Geometry check sheet. Reference: the model listing, model coordinates, mm. A direction names the side the tool comes from. Round coordinates to 2 decimals unless told otherwise and drop trailing zeros. Write each loop counter-clockwise with the first axis right and the second up, starting at its lowest first coordinate (ties: lowest second). Pieces come first, ordered by that corner, then holes. Notation, with made-up numbers: M 58,-15.5 L 67,-15.5 A21 cw 67,22.5 Z; hole C -32.5,53.25 d10. An arc over 180 degrees is marked long. Use a Markdown table: item, result.
```python
from build123d import *

# Parameters (mm, degrees)
ESQUISSE1_W             = 230
ESQUISSE1_H             = 270
BOSS_EXTRU_2_DEPTH      = 2.5
ENL_V_MAT_EXTRU_1_REACH = 405.102
ESQUISSE4_W             = 210
ESQUISSE4_H             = 23
ESQUISSE5_R             = 2
ENL_V_MAT_EXTRU_2_DEPTH = 2.5
ESQUISSE6_W             = 35
ESQUISSE6_H             = 8
ESQUISSE6_W_2           = 115
ESQUISSE6_H_2           = 25
ENL_V_MAT_EXTRU_3_DEPTH = 2.5
ESQUISSE7_W             = 29
ESQUISSE7_H             = 13
ENL_V_MAT_EXTRU_4_DEPTH = 2.5
ESQUISSE8_W             = 160
ESQUISSE8_H             = 2.5
BOSS_EXTRU_3_DEPTH      = 8
ESQUISSE9_R             = 2
ENL_V_MAT_EXTRU_5_DEPTH = 404.231037827
ESQUISSE11_R            = 2
ENL_V_MAT_EXTRU_6_DEPTH = 404.231037827


with BuildPart() as part:
    # Esquisse1 → Boss.-Extru.2 (new body)
    with BuildSketch(Plane.XY.offset(25)):
        with Locations((-102.459507472, 204.405925813)):
            Rectangle(ESQUISSE1_W, ESQUISSE1_H)
    extrude(amount=BOSS_EXTRU_2_DEPTH)

    # Esquisse4 → Enlèv. mat.-Extru.1 (cut, up to next)
    with BuildSketch(Plane.XY.offset(27.5), mode=Mode.PRIVATE) as enl_v_mat_extru_1_sk1:
        with Locations((-102.459507472, 87.905925813)):
            Rectangle(ESQUISSE4_W, ESQUISSE4_H)
    enl_v_mat_extru_1_tool1 = extrude(enl_v_mat_extru_1_sk1.sketch, amount=-ENL_V_MAT_EXTRU_1_REACH, mode=Mode.PRIVATE) & part.part
    add(enl_v_mat_extru_1_tool1.solids().sort_by_distance((-102.459507, 87.905926, 27.5))[0], mode=Mode.SUBTRACT)

    # Esquisse5 → Enlèv. mat.-Extru.2 (cut)
    with BuildSketch(Plane.XY.offset(27.5)):
        with Locations((-213.459507472, 73.405925813)):
            Circle(ESQUISSE5_R)
        with Locations((8.540492528, 73.405925813)):
            Circle(ESQUISSE5_R)
    extrude(amount=-ENL_V_MAT_EXTRU_2_DEPTH, mode=Mode.SUBTRACT)

    # Esquisse6 → Enlèv. mat.-Extru.3 (cut)
    with BuildSketch(Plane.XY.offset(27.5)):
        with Locations((-168.959507472, 249.405925813)):
            Rectangle(ESQUISSE6_W, ESQUISSE6_H)
        with Locations((-68.959507472, 240.905925813)):
            Rectangle(ESQUISSE6_W_2, ESQUISSE6_H_2)
    extrude(amount=-ENL_V_MAT_EXTRU_3_DEPTH, mode=Mode.SUBTRACT)

    # Esquisse7 → Enlèv. mat.-Extru.4 (cut)
    with BuildSketch(Plane.XY.offset(27.5)):
        with Locations((-131.959507472, 218.905925813)):
            Rectangle(ESQUISSE7_W, ESQUISSE7_H)
        with Locations((-183.959507472, 218.905925813)):
            Rectangle(ESQUISSE7_W, ESQUISSE7_H)
        with Locations((-79.959507472, 218.905925813)):
            Rectangle(ESQUISSE7_W, ESQUISSE7_H)
        with Locations((-27.959507472, 218.905925813)):
            Rectangle(ESQUISSE7_W, ESQUISSE7_H)
        with Locations((-131.959507472, 188.905925813)):
            Rectangle(ESQUISSE7_W, ESQUISSE7_H)
        with Locations((-79.959507472, 188.905925813)):
            Rectangle(ESQUISSE7_W, ESQUISSE7_H)
        with Locations((-27.959507472, 188.905925813)):
            Rectangle(ESQUISSE7_W, ESQUISSE7_H)
        with Locations((-131.959507472, 158.905925813)):
            Rectangle(ESQUISSE7_W, ESQUISSE7_H)
        with Locations((-79.959507472, 158.905925813)):
            Rectangle(ESQUISSE7_W, ESQUISSE7_H)
        with Locations((-27.959507472, 158.905925813)):
            Rectangle(ESQUISSE7_W, ESQUISSE7_H)
        with Locations((-131.959507472, 128.905925813)):
            Rectangle(ESQUISSE7_W, ESQUISSE7_H)
        with Locations((-79.959507472, 128.905925813)):
            Rectangle(ESQUISSE7_W, ESQUISSE7_H)
        with Locations((-27.959507472, 128.905925813)):
            Rectangle(ESQUISSE7_W, ESQUISSE7_H)
        with Locations((-183.959507472, 188.905925813)):
            Rectangle(ESQUISSE7_W, ESQUISSE7_H)
        with Locations((-183.959507472, 158.905925813)):
            Rectangle(ESQUISSE7_W, ESQUISSE7_H)
        with Locations((-183.959507472, 128.905925813)):
            Rectangle(ESQUISSE7_W, ESQUISSE7_H)
    extrude(amount=-ENL_V_MAT_EXTRU_4_DEPTH, mode=Mode.SUBTRACT)

    # Esquisse8 → Boss.-Extru.3 (add)
    with BuildSketch(Plane(origin=(0, 0, 25), x_dir=(-1, 0, 0), z_dir=(0, 0, -1))):
        with Locations((114.330010258, 199.655925813)):
            Rectangle(ESQUISSE8_W, ESQUISSE8_H)
    extrude(amount=BOSS_EXTRU_3_DEPTH)

    # Esquisse9 → Enlèv. mat.-Extru.5 (cut, through all)
    with BuildSketch(Plane.XY.offset(27.5)):
        with Locations((-209.959507472, 265.405925813)):
            Circle(ESQUISSE9_R)
    extrude(amount=-ENL_V_MAT_EXTRU_5_DEPTH, mode=Mode.SUBTRACT)

    # Esquisse11 → Enlèv. mat.-Extru.6 (cut, through all)
    with BuildSketch(Plane.XY.offset(27.5)):
        with Locations((5.040492528, 265.405925813)):
            Circle(ESQUISSE11_R)
    extrude(amount=-ENL_V_MAT_EXTRU_6_DEPTH, mode=Mode.SUBTRACT)


solid = part.part
```
Item 1: Material ranges on line 1 along Y through (x, z) = (-54, 25.5); line 2 along Z through (x, y) = (-205, 313.5); line 3 along Y through (x, z) = (-186, 17.5), recorded low to high. Write a range as from..to.
Outcome:
| item | result |
|---|---|
| line 1 | y = 69.41..76.41, 99.41..228.41, 253.41..339.41 |
| line 2 | z = 25..27.5 |
| line 3 | y = 198.41..200.91 |
Item 2: Go/stop test with a flat-tipped pin: pin 1 (6 mm diameter, centred on x = -10.5, z = 20.5, fed in from +Y). Record where the tip stops, or that it passes through.
Outcome:
| item | result |
|---|---|
| pin 1 | passes through |
Item 3: Cross-section at B-B, the plane y = 131.5. Record the cut outline in (x, z).
Outcome:
| item | result |
|---|---|
| outline | M -217.46,25 L -198.46,25 L -198.46,27.5 L -217.46,27.5 Z; M -169.46,25 L -146.46,25 L -146.46,27.5 L -169.46,27.5 Z; M -117.46,25 L -94.46,25 L -94.46,27.5 L -117.46,27.5 Z; M -65.46,25 L -42.46,25 L -42.46,27.5 L -65.46,27.5 Z; M -13.46,25 L 12.54,25 L 12.54,27.5 L -13.46,27.5 Z |
Item 4: Cross-section at C-C, the plane x = -3.5. Record the cut outline in (y, z), and give its area (4 significant figures).
Outcome:
| item | result |
|---|---|
| outline | M 69.41,25 L 76.41,25 L 76.41,27.5 L 69.41,27.5 Z; M 99.41,25 L 339.41,25 L 339.41,27.5 L 99.41,27.5 Z |
| area | 617.5 mm2 |
Item 5: Access from +Z, -Z, +X, -X, +Y, -Y to the whole of each face (thin tool, end or side, straight path). Record for faces 1 (the face through (-113, 198.406, 21)), 2 (the face through (-104, 206, 27.5)), 3 (the face through (-113, 200.906, 21)).
Outcome:
| item | result |
|---|---|
| face 1 | -Z, +X, -X, -Y |
| face 2 | +Z, +X, -X, +Y, -Y |
| face 3 | -Z, +X, -X, +Y |
Item 6: Cross-section at A-A, the plane x = -123. Count the separate pieces of the cut face and the enclosed holes in it, and give its area (3 significant figures).
Outcome:
| item | result |
|---|---|
| separate pieces | 7 |
| enclosed holes | 0 |
| area | 445 mm2 |
